```python
from build123d import *

# Parameters (mm, degrees)
F0_R     = 25.4
F0_R_2   = 7.62
F1_DEPTH = 2.54
F2_DEPTH = 63.5
F3_R     = 25.4
F3_R_2   = 7.62
F4_DEPTH = 2.54


with BuildPart() as f1:
    # F0 (on Top) → F1 (new body)
    with BuildSketch(Plane.XY):
        Circle(F0_R)
        Circle(F0_R_2, mode=Mode.SUBTRACT)
    extrude(amount=F1_DEPTH)

    # F0 (on Top) → F2 (join)
    with BuildSketch(Plane.XY):
        Circle(F0_R_2)
    extrude(amount=F2_DEPTH)

    # F3 (on face) → F4 (join)
    with BuildSketch(Plane.XY.offset(63.5)):
        Circle(F3_R)
        Circle(F3_R_2)
    extrude(amount=F4_DEPTH)


solid = f1.part
```
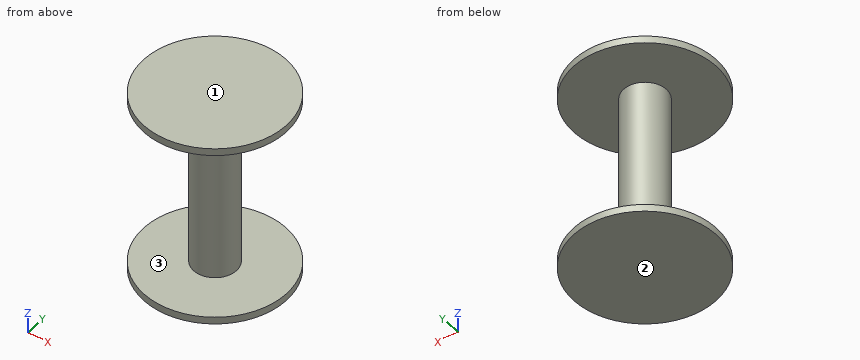
Model file for the job. Use its own axes, mm. Face numbers are marked on the shaded views. Coordinates: 2 decimals unless noted, no trailing zeros. Order: outer loops, then holes, each group sorted by start corner. A loop starts at its lowest first (then second) coordinate and runs counter-clockwise, first axis right, second up. Notation, with made-up numbers: (-15, 67.5) -> (44, 67.5) arc R18 cw to (44, 94.5) -> close; hole circle Ø1 at (2, 36.5). An arc over 180 degrees is marked (long way). Return JSON: item names as keys, results as strings.
Item 1: Wall check: line 1 along Z through (x, y) = (8.5, 23); line 2 along X through (y, z) = (4, 37); line 3 along Y through (x, z) = (2, 39). Give the ranges that are in metal, low to high. Write a range as from..to.
Model answer:
{"line 1": "z = 0..2.54, 63.5..66.04", "line 2": "x = -6.49..6.49", "line 3": "y = -7.35..7.35"}
Item 2: Pin check, flat tips, straight feed: P1, Ø2, axis at x = 4.5, z = 50, coming from the +Y side; P2, Ø3, axis at y = -5, z = 20.5, coming from the +X side; P3, Ø5, axis at y = -0.5, z = 24, coming from the -X side. Stop position of each tip, or through.
Model answer:
{"P1": "stops at y = 6.77", "P2": "stops at x = 6.77", "P3": "stops at x = -7.62"}
Item 3: Slice it at A-A (x = 10.5). Write the cut outline in (y, z), then the cut area to 3 significant figures.
Model answer:
{"outline": "(-23.13, 0) -> (23.13, 0) -> (23.13, 2.54) -> (-23.13, 2.54) -> close; (-23.13, 63.5) -> (23.13, 63.5) -> (23.13, 66.04) -> (-23.13, 66.04) -> close", "area": "235 mm²"}
Item 4: Mould opens along Z. For the marked faces 1, 2 and 3 say: pulls with the +Z half, pulls with the -Z half, needs draft (parallel to the pull), parting line crosses it, or undercut.
Model answer:
{"face 1": "pulls with the +Z half", "face 2": "pulls with the -Z half", "face 3": "undercut"}
Item 5: Slice it at D-D (z = 56). Write the cut outline in (x, y), then the cut area to 3 significant figures.
Model answer:
{"outline": "circle Ø15.24 at (0, 0)", "area": "182 mm²"}
Item 6: Slice it at B-B (y = 0). Write the cut outline in (x, z).
Model answer:
{"outline": "(-25.4, 0) -> (25.4, 0) -> (25.4, 2.54) -> (7.62, 2.54) -> (7.62, 63.5) -> (25.4, 63.5) -> (25.4, 66.04) -> (-25.4, 66.04) -> (-25.4, 63.5) -> (-7.62, 63.5) -> (-7.62, 2.54) -> (-25.4, 2.54) -> close"}
